The drawing under review shows one solid part. Ordinate dimensions are in mm from its lowest x, y, z. A direction names the side the tool comes from. Round coordinates to 2 decimals unless told otherwise and drop trailing zeros. Write each loop counter-clockwise with the first axis right and the second up, starting at its lowest first coordinate (ties: lowest second). Pieces come first, ordered by that corner, then holes. Notation, with made-up numbers: M 10.5,-39.75 L 63.5,-39.75 A20 ccw 63.5,-32.75 Z; hole C -27.5,87.25 d11. An arc over 180 degrees is marked long. One line per item, written item: value. Start each with the question number.
1) Mouldability with a two-part tool opening along X and no side actions: class the marked faces 1, 2 and 3 as +X half, -X half, draft (parallel to the pull), parting line (faces both ways), or undercut.
2) For P1, Ø1.5, axis at x = 11.5, z = 13, coming from the +Y side; P2, Ø1.5, axis at x = 58, z = 8.5, coming from the -Y side; P3, Ø4, axis at x = 32, z = 14.5, coming from the +Y side, all flat-tipped, find the tip position at first contact; note any pin that passes through.
3) Tool access review of the marked faces 4 and 5: name each direction out of +Z, -Z, +X, -X, +Y, -Y from which nothing blocks a thin tool from reaching the whole face with its end or side.
4) Take a section at D-D, the plane y = 61. Write out the cut boundary in (x, z) (1 decimal).
5) Wall thickness on probe 1 along Y at (x, z) = (21, 2.75); probe 2 along Y at (x, z) = (50.5, 13.5); probe 3 along X at (y, z) = (103.5, 2.25) (1 decimal): over which ranges is each line inside the solid? List them lowest first.
6) Take a section at C-C, the plane x = 17. Write out the cut boundary in (y, z) (1 decimal).
7) Take a section at B-B, the plane z = 9.5. Write out the cut boundary in (x, y) (1 decimal), and give its area (3 significant figures).
8) Take a section at A-A, the plane x = 40.5. Write out the cut boundary in (y, z) (1 decimal).
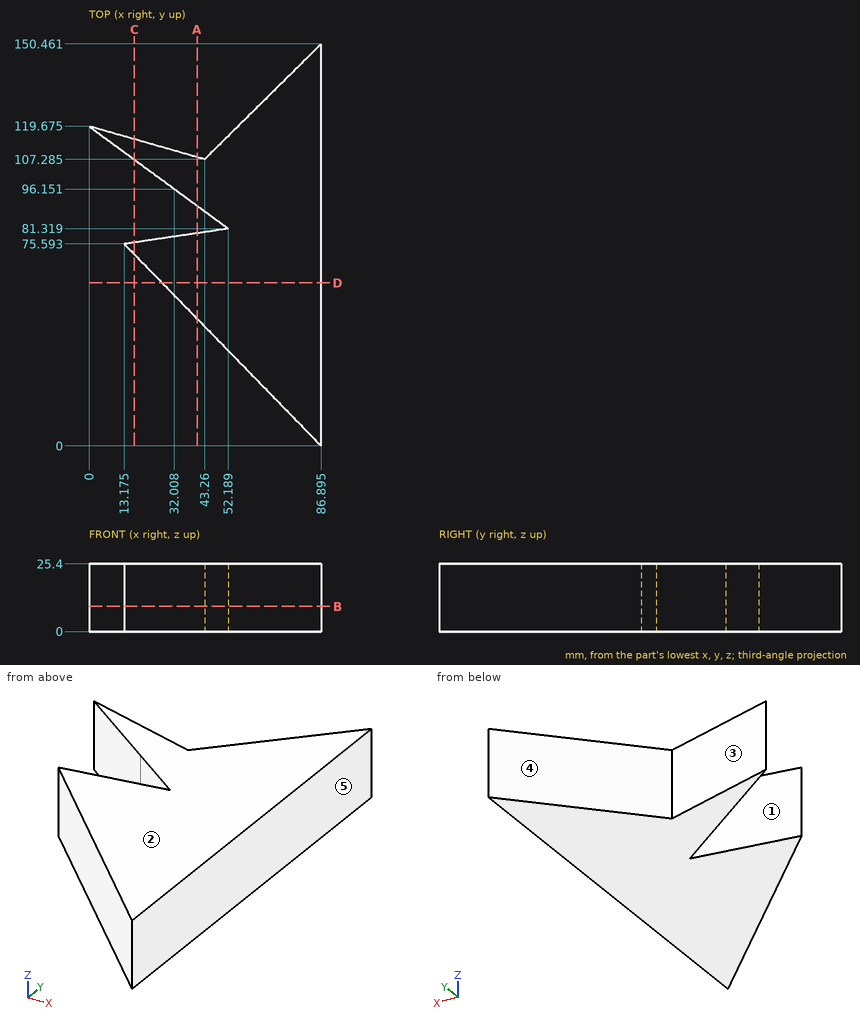
Checked values:
1. face 1: -X half
1. face 2: draft
1. face 3: undercut
2. P1: stops at y = 116.6
2. P2: stops at y = 28.86
2. P3: stops at y = 111.08
3. face 4: +Z, -Z, +Y
3. face 5: +Z, -Z, +X, +Y, -Y
4. outline: M 27.4,0 L 86.9,0 L 86.9,25.4 L 27.4,25.4 Z
5. probe 1: y = 67.57 to 76.74, 104.24 to 113.66
5. probe 2: y = 37.32 to 81.07, 82.56 to 114.45
5. probe 3: x = 22 to 86.9
6. outline: M 71.7,0 L 76.2,0 L 76.2,25.4 L 71.7,25.4 Z; M 107.2,0 L 114.8,0 L 114.8,25.4 L 107.2,25.4 Z
7. outline: M 0,119.7 L 52.2,81.3 L 13.2,75.6 L 86.9,0 L 86.9,150.5 L 43.3,107.3 Z
7. area: 5,560 mm2
8. outline: M 47.6,0 L 79.6,0 L 79.6,25.4 L 47.6,25.4 Z; M 89.9,0 L 108.1,0 L 108.1,25.4 L 89.9,25.4 Z
